Could you check a few things on this model? Use its own coordinates, in mm. A direction names the side the tool comes from. Give positions to 0.01 mm unless a question says otherwise; leave off trailing zeros. Order: outer loops, then holes, each group sorted by start corner. A loop starts at its lowest first (then second) coordinate and runs counter-clockwise, first axis right, second up. Notation, with made-up numbers: (-19.5, 10) - (36.5, 10) arc R20 ccw to (36.5, 46) - close; hole circle Ø7 at (65, 64). An arc over 180 degrees is marked (long way). One line per question, with ' | ' between items. Start each with the question number.
1. Imagine slicing it at A-A (y = -7). Please give me the cut outline in (x, z) (3 decimals).
2. Which directions (+Z, -Z, +X, -X, +Y, -Y) give clear straight access to the entire face, cutting with the end or side of a thin tool? Please do faces 1 (the flat face through (-1.02, -8.12, 0.13)), 2 (the flat face through (9.525, 0, 0)).
3. For P1, Ø1.5, axis at x = -2, z = -1, coming from the +Y side; P2, Ø1, axis at x = 3.5, y = 2, coming from the -Z side, each with a flat end and sliding along its axis, tell me the tip position at first contact or that it passes through.
4. Imagine slicing it at C-C (z = 2.25). Please give me the cut outline in (x, y) (3 decimals), and give its area (3 significant figures).
5. I need wall thicknesses on probe 1 along Y at (x, z) = (-1.25, -0.75); probe 2 along Y at (x, z) = (3, 2); probe 3 along Y at (x, z) = (0.75, 2). Which ranges of each line are inside material? Lowest first, please. Write a range as from..to.
6. Imagine slicing it at B-B (x = 4.25). Please give me the cut outline in (y, z) (3 decimals), and give its area (3 significant figures).
7. Imagine slicing it at D-D (x = -7). Please give me the cut outline in (y, z) (3 decimals).
8. If we mould it in two halves opening along Y, with no side actions, what happens to faces 3 (the flat face through (-9.525, 0, 0)), 4 (the flat face through (-5.56, -7.79, 0.13)), 5 (the flat face through (-0.17, -8.23, 0.13))? For each: released by +Y, released by -Y, zero draft, split by the parting line, or undercut.
```python
from build123d import *

# Parameters (mm, degrees)
SKETCH1_R         = 6.35
EXTRUDE1_DEPTH    = 9.525
SKETCH2_OUTSIDE_W = 28.006
SKETCH2_OUTSIDE_H = 30.954
SKETCH2_OUTSIDE_R = 10.715625
EXTRUDE2_DEPTH    = 24.970724332
EXTRUDE3_DEPTH    = 24.842247045


with BuildPart() as part:
    # Sketch1 → Extrude1 (new, symmetric)
    with BuildSketch(Plane.XY):
        Polygon((0, 10.998522628), (-9.525, 5.499261314), (-9.525, -5.499261314), (0, -10.998522628), (9.525, -5.499261314), (9.525, 5.499261314), align=None)
        with Locations(Location((0, 0, 0), (0, 0, 180))):
            Circle(SKETCH1_R, mode=Mode.SUBTRACT)
    extrude(amount=EXTRUDE1_DEPTH, both=True)

    # Sketch2 outside → Extrude2 (cut, through all)
    with BuildSketch(Plane.XY.offset(9.525)):
        Rectangle(SKETCH2_OUTSIDE_W, SKETCH2_OUTSIDE_H)
        Circle(SKETCH2_OUTSIDE_R, mode=Mode.SUBTRACT)
    extrude(amount=-EXTRUDE2_DEPTH, mode=Mode.SUBTRACT)

    # Sketch3 → Extrude3 (cut, through all)
    with BuildSketch(Plane.XY.offset(9.525)):
        Polygon((3.437038321, -1.984375), (-1.325461679, -10.233266971), (-2.012869343, -9.836391971), (2.749630657, -1.5875), align=None)
    extrude(amount=-EXTRUDE3_DEPTH, mode=Mode.SUBTRACT)


solid = part.part
```
Results found:
1) outline: (-6.926, -9.525) - (-0.375, -9.525) - (-0.375, 9.525) - (-6.926, 9.525) - close; (0.541, -9.525) - (6.926, -9.525) - (6.926, 9.525) - (0.541, 9.525) - close
2) face 1: +Z, -Z | face 2: +Z, -Z, +X, +Y, -Y
3) P1: stops at y = 10.28 | P2: passes through
4) outline: (-9.525, -4.909) arc R10.716 ccw to (-9.014, -5.794) - (-2.013, -9.836) - (0, -6.35) arc R6.35 cw (long way) to (0.959, -6.277) - (-1.325, -10.233) - (-0.511, -10.703) arc R10.716 ccw to (0.511, -10.703) - (9.014, -5.794) arc R10.716 ccw to (9.525, -4.909) - (9.525, 4.909) arc R10.716 ccw to (9.014, 5.794) - (0.511, 10.703) arc R10.716 ccw to (-0.511, 10.703) - (-9.014, 5.794) arc R10.716 ccw to (-9.525, 4.909) - close | area: 183 mm2
5) probe 1: y = -10.28..-10.1, -8.52..-6.23, 6.23..10.28 | probe 2: y = -9.27..-5.6, 5.6..9.27 | probe 3: y = -10.57..-6.64, 6.31..10.57
6) outline: (-8.545, -9.525) - (-4.718, -9.525) - (-4.718, 9.525) - (-8.545, 9.525) - close; (4.718, -9.525) - (8.545, -9.525) - (8.545, 9.525) - (4.718, 9.525) - close | area: 146 mm2
7) outline: (-6.957, -9.525) - (6.957, -9.525) - (6.957, 9.525) - (-6.957, 9.525) - close
8) face 3: zero draft | face 4: released by -Y | face 5: undercut
